Geometry: final body of the model. Coordinates: model frame, mm. A direction names the side the tool comes from. Coordinates: 2 decimals unless noted, no trailing zeros. Order: outer loops, then holes, each group sorted by start corner. A loop starts at its lowest first (then second) coordinate and runs counter-clockwise, first axis right, second up. Notation, with made-up numbers: (-10.5, -39) -> (32.5, -39) arc R23 cw to (32.5, -7) -> close; hole circle Ø11 at (41.25, 1). An arc over 180 degrees is marked (long way). Answer in a Markdown table with one row per item. Add a question column.
1) Ray query, line 1 (Y direction, x = 0, z = 9.5); line 2 (Y direction, x = 3.5, z = 27); line 3 (Z direction, x = 0, y = 1.5). Return the intervals inside material, ascending. Write a range as from..to.
2) Contact query for flat-ended pins moving along their axis: P1, Ø8, axis at y = 8, z = 13, coming from the -X side; P2, Ø12, axis at y = -6, z = 32.5, coming from the -X side; P3, Ø4, axis at x = 2, y = 7, coming from the +Z side; P4, Ø1.8, axis at x = 4.5, y = 11.5, coming from the -Z side. Output: stop coordinate, or through.
3) Set-up query: faces 1 (the face through (5, -12, 50)), 2 (the face through (-2, 2, 25)), 3 (the face through (-5, -12, 50)). Return all of +Z, -Z, +X, -X, +Y, -Y with unobstructed straight access to the full face (end or side cutting, diameter ignored); none if empty.
4) Section query A-A on z = 6. Return the cut outline in (x, y).
5) Pull-direction query (Z, two-part tool) for faces 4 (the face through (-3, 2, 27)), 5 (the face through (0.19, 8.635, 42.274)), 6 (the face through (-6.25, 0, 47)), 7 (the face through (0, 9, 53)); classes: +Z half, -Z half, draft (parallel to the pull), parting line (faces both ways), or undercut.
```python
from build123d import *

# Parameters (mm, degrees)
SKETCH1_R           = 6.25
BOSS_EXTRUDE1_DEPTH = 50
SKETCH8_R           = 2.15
CUT_EXTRUDE3_DEPTH  = 25
CUT_EXTRUDE4_DEPTH  = 3.5
SKETCH10_W          = 12.5
SKETCH10_H          = 25
BOSS_EXTRUDE2_DEPTH = 3
SKETCH12_W          = 7.267551801
SKETCH12_H          = 25
SKETCH12_W_2        = 9.375486859
CUT_EXTRUDE5_DEPTH  = 54
SKETCH13_R          = 2.15
CUT_EXTRUDE6_DEPTH  = 25.5
SKETCH14_R          = 6.25
BOSS_EXTRUDE3_DEPTH = 5
CHAMFER1_SIZE       = 1


with BuildPart() as part:
    # Sketch1 → Boss-Extrude1 (new body)
    with BuildSketch(Plane.XY):
        Circle(SKETCH1_R)
    extrude(amount=BOSS_EXTRUDE1_DEPTH)

    # Sketch8 → Cut-Extrude3 (cut)
    with BuildSketch(Plane(origin=(0, 0, 0), x_dir=(-1, 0, 0), z_dir=(0, 0, -1))):
        Circle(SKETCH8_R)
    extrude(amount=-CUT_EXTRUDE3_DEPTH, mode=Mode.SUBTRACT)

    # Sketch9 → Cut-Extrude4 (cut)
    with BuildSketch(Plane(origin=(0, 0, 25), x_dir=(-1, 0, 0), z_dir=(0, 0, -1))):
        Polygon((4.156921938, 0), (2.078460969, 3.6), (-2.078460969, 3.6), (-4.156921938, 0), (-2.078460969, -3.6), (2.078460969, -3.6), align=None)
    extrude(amount=-CUT_EXTRUDE4_DEPTH, mode=Mode.SUBTRACT)

    # Sketch10 → Boss-Extrude2 (add)
    with BuildSketch(Plane.XY.offset(50)):
        Rectangle(SKETCH10_W, SKETCH10_H)
    extrude(amount=BOSS_EXTRUDE2_DEPTH)

    # Sketch11 → Revolve1 (revolve)
    with BuildSketch(Plane(origin=(0, 0, 0), x_dir=(0, 0, -1), z_dir=(1, 0, 0))):
        Polygon((-50, 12.5), (-37.5, 6.25), (-37.5, 0), (-50, 0), align=None)
    revolve(axis=Axis((0, 0, 63.541170981), (0, 0, 1)))

    # Sketch12 → Cut-Extrude5 (cut, through all)
    with BuildSketch(Plane.XY.offset(53)):
        with Locations((-9.883775901, 0)):
            Rectangle(SKETCH12_W, SKETCH12_H)
        with Locations((10.937743429, 0)):
            Rectangle(SKETCH12_W_2, SKETCH12_H)
    extrude(amount=-CUT_EXTRUDE5_DEPTH, mode=Mode.SUBTRACT)

    # Sketch13 → Cut-Extrude6 (cut, through all)
    with BuildSketch(Plane(origin=(0, 0, 28.5), x_dir=(-1, 0, 0), z_dir=(0, 0, -1))):
        Circle(SKETCH13_R)
    extrude(amount=-CUT_EXTRUDE6_DEPTH, mode=Mode.SUBTRACT)

    # Sketch14 → Boss-Extrude3 (add)
    with BuildSketch(Plane.XY.offset(53)):
        Circle(SKETCH14_R)
    extrude(amount=BOSS_EXTRUDE3_DEPTH)

    # Chamfer1
    chamfer1_edges = [part.edges().sort_by_distance(p)[0] for p in [
        (-6.25, 0, 58),
    ]]
    chamfer(chamfer1_edges, length=CHAMFER1_SIZE)


solid = part.part
```
Result:
| question | item | result |
|---|---|---|
| 1 | line 1 | -6.25..-2.15, 2.15..6.25 |
| 1 | line 2 | -5.18..-1.14, 1.14..5.18 |
| 1 | line 3 | 53..58 |
| 2 | P1 | x = -4.8 |
| 2 | P2 | x = -6.25 |
| 2 | P3 | z = 57.97 |
| 2 | P4 | z = 47.9 |
| 3 | face 1 | -Z, +X, -Y |
| 3 | face 2 | none |
| 3 | face 3 | -Z, -X, -Y |
| 4 | outline | circle Ø12.5 at (0, 0); hole circle Ø4.3 at (0, 0) |
| 5 | face 4 | undercut |
| 5 | face 5 | -Z half |
| 5 | face 6 | draft |
| 5 | face 7 | +Z half |
